from build123d import *

# Parameters (mm, degrees)
BOSS_EXTRUDE1_DEPTH            = 508
SKETCH2_W                      = 175.72130466
SKETCH2_H                      = 449.160798253
CUT_EXTRUDE1_DEPTH             = 76.2
SKETCH3_W                      = 304.8
SKETCH3_H                      = 203.2
CUT_EXTRUDE3_DEPTH             = 50.8
SHELL2_START                   = 27.94
SHELL2_DEPTH                   = 452.12
SHELL2_2_DEPTH                 = 45.72
SHELL2_START_2                 = 434.34
SHELL2_3_DEPTH                 = 45.72
FILLET1_R                      = 7.62
CUT_EXTRUDE4_REACH             = 965.862
CUT_EXTRUDE4_DIRECTION_2_DEPTH = 97.536
CUT_EXTRUDE5_REACH             = 832.247


# Read off the part's stored shape, not the designer's step: Shell2
with BuildPart() as part:
    # Sketch1 → Boss-Extrude1 (new body)
    with BuildSketch(Plane.XY):
        Polygon((508, 0), (508, 371.248348728), (279.4, 371.248348728), (83.128822626, 711.2), (0, 711.2), (0, 0), align=None)
    extrude(amount=BOSS_EXTRUDE1_DEPTH)

    # Sketch2 → Cut-Extrude1 (cut)
    with BuildSketch(Plane(origin=(0, 371.248348728, 0), x_dir=(1, 0, 0), z_dir=(0, 1, 0))):
        with Locations((387.505332687, -250.48614125)):
            Rectangle(SKETCH2_W, SKETCH2_H)
    extrude(amount=-CUT_EXTRUDE1_DEPTH, mode=Mode.SUBTRACT)

    # Sketch3 → Cut-Extrude3 (cut)
    with BuildSketch(Plane(origin=(370.305250556, 213.795836091, 0), x_dir=(0, 0, -1), z_dir=(0.8660254037844397, 0.49999999999999806, 0))):
        with Locations((-254, 371.152855858)):
            Rectangle(SKETCH3_W, SKETCH3_H)
    extrude(amount=-CUT_EXTRUDE3_DEPTH, mode=Mode.SUBTRACT)

    # Shell2 outline → Shell2 (cut)
    with BuildSketch(Plane.XY.offset(SHELL2_START)):
        Polygon((27.94, 27.94), (480.06, 27.94), (480.06, 267.108348728), (271.704680357, 267.108348728), (271.704680357, 343.308348728), (263.268833479, 343.308348728), (225.302072845, 409.068707145), (205.504732114, 397.638707145), (191.534732114, 421.835456927), (89.934732114, 597.811818976), (75.964732114, 622.008568757), (95.762072845, 633.438568757), (66.997656105, 683.26), (27.94, 683.26), align=None)
    extrude(amount=SHELL2_DEPTH, mode=Mode.SUBTRACT)

    # Shell2 2 outline → Shell2 2 (cut)
    with BuildSketch(Plane.XY.offset(SHELL2_START)):
        Polygon((225.302072845, 409.068707145), (95.762072845, 633.438568757), (75.964732114, 622.008568757), (89.934732114, 597.811818976), (191.534732114, 421.835456927), (205.504732114, 397.638707145), align=None)
    extrude(amount=SHELL2_2_DEPTH, mode=Mode.SUBTRACT)

    # Shell2 3 outline → Shell2 3 (cut)
    with BuildSketch(Plane.XY.offset(SHELL2_START_2)):
        Polygon((225.302072845, 409.068707145), (95.762072845, 633.438568757), (75.964732114, 622.008568757), (89.934732114, 597.811818976), (191.534732114, 421.835456927), (205.504732114, 397.638707145), align=None)
    extrude(amount=SHELL2_3_DEPTH, mode=Mode.SUBTRACT)

    # Fillet1
    fillet1_edges = [part.edges().sort_by_distance(p)[0] for p in [
        (508, 185.624174364, 0),
        (393.7, 371.248348728, 508),
        (83.128822626, 711.2, 254),
        (508, 371.248348728, 254),
        (181.264411313, 541.224174364, 508),
        (41.564411313, 711.2, 508),
        (508, 185.624174364, 508),
        (41.564411313, 711.2, 0),
        (181.264411313, 541.224174364, 0),
        (393.7, 371.248348728, 0),
    ]]
    fillet(fillet1_edges, radius=FILLET1_R)

    # Cut-Extrude4: up to this face of the body (flat: up to its plane)
    cut_extrude4_end = Plane(part.part.faces().sort_by_distance((162.73177737, 522.523637951, 101.6))[0])
    # Sketch6 → Cut-Extrude4 (cut, up to the picked face)
    with BuildSketch(Plane(origin=(0, 0, 406.4), x_dir=(-1, 0, 0), z_dir=(0, 0, -1)), mode=Mode.PRIVATE) as cut_extrude4_sk1:
        Polygon((-109.711824261, 652.442307464), (-240.02087993, 424.214985446), (-218.44952186, 411.898566558), (-97.827125151, 645.656599669), align=None)
    cut_extrude4_tool1 = split(extrude(cut_extrude4_sk1.sketch, amount=CUT_EXTRUDE4_REACH, mode=Mode.PRIVATE), bisect_by=cut_extrude4_end, keep=Keep.BOTH, mode=Mode.PRIVATE)
    add(cut_extrude4_tool1.solids().sort_by(Axis((172.556766, 522.406417, 406.4), (0, 0, -1)))[0], mode=Mode.SUBTRACT)

    # Sketch6 → Cut-Extrude4 direction 2 (cut)
    with BuildSketch(Plane(origin=(0, 0, 406.4), x_dir=(-1, 0, 0), z_dir=(0, 0, -1))):
        Polygon((-109.711824261, 652.442307464), (-240.02087993, 424.214985446), (-218.44952186, 411.898566558), (-97.827125151, 645.656599669), align=None)
    extrude(amount=-CUT_EXTRUDE4_DIRECTION_2_DEPTH, mode=Mode.SUBTRACT)

    # Sketch10 → Cut-Extrude5 (cut, up to next)
    with BuildSketch(Plane(origin=(0, 295.048348728, 0), x_dir=(1, 0, 0), z_dir=(0, 1, 0)), mode=Mode.PRIVATE) as cut_extrude5_sk1:
        with BuildLine():
            Line((384.681985017, -385.451435914), (385.481985017, -385.451435914))
            ThreePointArc((385.481985017, -385.451435914), (386.896198579, -386.037222352), (387.481985017, -387.451435914))
            Line((387.481985017, -387.451435914), (387.481985017, -408.951435914))
            ThreePointArc((387.481985017, -408.951435914), (386.896198579, -410.365649476), (385.481985017, -410.951435914))
            Line((385.481985017, -410.951435914), (384.681985017, -410.951435914))
            ThreePointArc((384.681985017, -410.951435914), (383.267771454, -410.365649476), (382.681985017, -408.951435914))
            Line((382.681985017, -408.951435914), (382.681985017, -387.451435914))
            ThreePointArc((382.681985017, -387.451435914), (383.267771454, -386.037222352), (384.681985017, -385.451435914))
        make_face()
    cut_extrude5_tool1 = extrude(cut_extrude5_sk1.sketch, amount=-CUT_EXTRUDE5_REACH, mode=Mode.PRIVATE) & part.part
    # Sketch10 → Cut-Extrude5 (cut, up to next)
    with BuildSketch(Plane(origin=(0, 295.048348728, 0), x_dir=(1, 0, 0), z_dir=(0, 1, 0)), mode=Mode.PRIVATE) as cut_extrude5_sk2:
        with BuildLine():
            Line((385.481985017, -312.438871317), (384.681985017, -312.438871317))
            ThreePointArc((384.681985017, -312.438871317), (383.267771454, -311.853084879), (382.681985017, -310.438871317))
            Line((382.681985017, -310.438871317), (382.681985017, -288.938871317))
            ThreePointArc((382.681985017, -288.938871317), (383.267771454, -287.524657755), (384.681985017, -286.938871317))
            Line((384.681985017, -286.938871317), (385.481985017, -286.938871317))
            ThreePointArc((385.481985017, -286.938871317), (386.896198579, -287.524657755), (387.481985017, -288.938871317))
            Line((387.481985017, -288.938871317), (387.481985017, -310.438871317))
            ThreePointArc((387.481985017, -310.438871317), (386.896198579, -311.853084879), (385.481985017, -312.438871317))
        make_face()
    cut_extrude5_tool2 = extrude(cut_extrude5_sk2.sketch, amount=-CUT_EXTRUDE5_REACH, mode=Mode.PRIVATE) & part.part
    # Sketch10 → Cut-Extrude5 (cut, up to next)
    with BuildSketch(Plane(origin=(0, 295.048348728, 0), x_dir=(1, 0, 0), z_dir=(0, 1, 0)), mode=Mode.PRIVATE) as cut_extrude5_sk3:
        with BuildLine():
            Line((385.481985017, -213.92630672), (384.681985017, -213.92630672))
            ThreePointArc((384.681985017, -213.92630672), (383.267771454, -213.340520282), (382.681985017, -211.92630672))
            Line((382.681985017, -211.92630672), (382.681985017, -190.42630672))
            ThreePointArc((382.681985017, -190.42630672), (383.267771454, -189.012093158), (384.681985017, -188.42630672))
            Line((384.681985017, -188.42630672), (385.481985017, -188.42630672))
            ThreePointArc((385.481985017, -188.42630672), (386.896198579, -189.012093158), (387.481985017, -190.42630672))
            Line((387.481985017, -190.42630672), (387.481985017, -211.92630672))
            ThreePointArc((387.481985017, -211.92630672), (386.896198579, -213.340520282), (385.481985017, -213.92630672))
        make_face()
    cut_extrude5_tool3 = extrude(cut_extrude5_sk3.sketch, amount=-CUT_EXTRUDE5_REACH, mode=Mode.PRIVATE) & part.part
    # Sketch10 → Cut-Extrude5 (cut, up to next)
    with BuildSketch(Plane(origin=(0, 295.048348728, 0), x_dir=(1, 0, 0), z_dir=(0, 1, 0)), mode=Mode.PRIVATE) as cut_extrude5_sk4:
        with BuildLine():
            Line((385.481985017, -115.413742123), (384.681985017, -115.413742123))
            ThreePointArc((384.681985017, -115.413742123), (383.267771454, -114.827955685), (382.681985017, -113.413742123))
            Line((382.681985017, -113.413742123), (382.681985017, -91.913742123))
            ThreePointArc((382.681985017, -91.913742123), (383.267771454, -90.499528561), (384.681985017, -89.913742123))
            Line((384.681985017, -89.913742123), (385.481985017, -89.913742123))
            ThreePointArc((385.481985017, -89.913742123), (386.896198579, -90.499528561), (387.481985017, -91.913742123))
            Line((387.481985017, -91.913742123), (387.481985017, -113.413742123))
            ThreePointArc((387.481985017, -113.413742123), (386.896198579, -114.827955685), (385.481985017, -115.413742123))
        make_face()
    cut_extrude5_tool4 = extrude(cut_extrude5_sk4.sketch, amount=-CUT_EXTRUDE5_REACH, mode=Mode.PRIVATE) & part.part
    add(cut_extrude5_tool1.solids().sort_by_distance((385.081985, 295.048349, 398.201436))[0], mode=Mode.SUBTRACT)
    add(cut_extrude5_tool2.solids().sort_by_distance((385.081985, 295.048349, 299.688871))[0], mode=Mode.SUBTRACT)
    add(cut_extrude5_tool3.solids().sort_by_distance((385.081985, 295.048349, 201.176307))[0], mode=Mode.SUBTRACT)
    add(cut_extrude5_tool4.solids().sort_by_distance((385.081985, 295.048349, 102.663742))[0], mode=Mode.SUBTRACT)


solid = part.part
Check sheet for the modelled part. Datum: model origin and axes. Units: mm. A direction names the side the tool comes from. Round coordinates to 2 decimals unless told otherwise and drop trailing zeros. Order: outer loops, then holes, each group sorted by start corner. A loop starts at its lowest first (then second) coordinate and runs counter-clockwise, first axis right, second up.
(1) Draft check along Z on faces 1 (the flat face through (250, 0, 250)), 2 (the flat face through (191, 279, 508)), 3 (the flat face through (150, 516, 73.66)). Enter one of: pulls with the +Z half, pulls with the -Z half, needs draft (parallel to the pull), parting line crosses it, or undercut.
(2) Go/stop test with flat-tipped pins: P1, Ø1, axis at x = 432, z = 272.5, coming from the +Y side; P2, Ø1, axis at y = 585.5, z = 136, coming from the +X side. Record where each tip stops, or that it passes through.
(3) Cross-section at B-B, the plane x = 368. Enter the section's corners in (y, z).
(4) Cross-section at A-A, the plane y = 226.5. Enter the section's corners in (x, z), and give its area (3 significant figures).
(5) Scan lines: probe 1 along X at (y, z) = (305, 397); probe 2 along Z at (x, y) = (326, 137.5); probe 3 along Y at (x, z) = (355, 239). Record each from-to range of solid material in increasing order.
(6) Access from +Z, -Z, +X, -X, +Y, -Y to the whole of each face (thin tool, end or side, straight path). Record for faces 4 (the flat face through (382.682, 281, 300)), 5 (the flat face through (480, 371.248, 198)), 6 (the flat face through (173.95, 539.93, 434.06)).
Check sheet entries:
1. face 1: needs draft
1. face 2: pulls with the +Z half
1. face 3: undercut
2. P1: stops at y = 295.05
2. P2: stops at x = 27.94
3. outline: (0, 0) - (363.63, 0) arc R7.62 ccw to (371.25, 7.62) - (371.25, 25.91) - (295.05, 25.91) - (295.05, 475.07) - (371.25, 475.07) - (371.25, 500.38) arc R7.62 ccw to (363.63, 508) - (0, 508) - close; hole (27.94, 27.94) - (267.11, 27.94) - (267.11, 480.06) - (27.94, 480.06) - close
4. outline: (0, 0) - (500.38, 0) arc R7.62 ccw to (508, 7.62) - (508, 500.38) arc R7.62 ccw to (500.38, 508) - (0, 508) - close; hole (27.94, 27.94) - (480.06, 27.94) - (480.06, 480.06) - (27.94, 480.06) - close
4. area: 53,600 mm2
5. probe 1: x = 0 to 27.94, 271.7 to 299.64, 475.37 to 508
5. probe 2: z = 0 to 27.94, 480.06 to 508
5. probe 3: y = 0 to 27.94, 267.11 to 295.05
6. face 4: +Y
6. face 5: +Z, -Z, +X, +Y
6. face 6: none
